Check sheet for the modelled part. Datum: model origin and axes. Units: mm. Face numbers are marked on the shaded views. A direction names the side the tool comes from. Round coordinates to 2 decimals unless told otherwise and drop trailing zeros. Write each loop counter-clockwise with the first axis right and the second up, starting at its lowest first coordinate (ties: lowest second). Pieces come first, ordered by that corner, then holes. Notation, with made-up numbers: (-21, -16.5) -> (31, -16.5) arc R36 cw to (31, 18.5) -> close; hole circle Ø11 at (18.5, 81). An arc over 180 degrees is marked (long way). Write item = value, one per line.
from build123d import *

# Parameters (mm, degrees)
SKETCH1_W           = 177.8
SKETCH1_H           = 50.8
BOSS_EXTRUDE2_DEPTH = 101.6
SKETCH5_W           = 101.6
SKETCH5_H           = 50.8
BOSS_EXTRUDE3_DEPTH = 76.2
BOSS_EXTRUDE4_DEPTH = 50.8
BOSS_EXTRUDE5_REACH = 103.6
SKETCH6_W           = 101.6
SKETCH6_H           = 50.8


with BuildPart() as part:
    # Sketch1 → Boss-Extrude2 (new body)
    with BuildSketch(Plane.XY):
        with Locations((88.9, 25.4)):
            Rectangle(SKETCH1_W, SKETCH1_H)
    extrude(amount=-BOSS_EXTRUDE2_DEPTH)

    # Sketch5 → Boss-Extrude3 (add)
    with BuildSketch(Plane(origin=(0, 0, 0), x_dir=(0, 0, -1), z_dir=(1, 0, 0))):
        with Locations((50.8, 76.2)):
            Rectangle(SKETCH5_W, SKETCH5_H)
    extrude(amount=BOSS_EXTRUDE3_DEPTH)

    # Sketch4 → Boss-Extrude4 (add)
    with BuildSketch(Plane(origin=(0, 50.8, 0), x_dir=(1, 0, 0), z_dir=(0, 1, 0))):
        Polygon((76.2, 50.8), (76.2, 0), (177.8, 50.8), (177.8, 101.6), (177.395806452, 101.6), (177.395806452, 50.8), align=None)
    extrude(amount=BOSS_EXTRUDE4_DEPTH)

    # Sketch6 → Boss-Extrude5 (add, up to next)
    with BuildSketch(Plane(origin=(76.2, 101.6, -101.6), x_dir=(1, 0, 0), z_dir=(0, 0, 1)), mode=Mode.PRIVATE) as boss_extrude5_sk1:
        with Locations((50.8, -25.4)):
            Rectangle(SKETCH6_W, SKETCH6_H)
    boss_extrude5_tool1 = extrude(boss_extrude5_sk1.sketch, amount=BOSS_EXTRUDE5_REACH, mode=Mode.PRIVATE) - part.part
    add(boss_extrude5_tool1.solids().sort_by_distance((127, 76.2, -101.6))[0])


solid = part.part
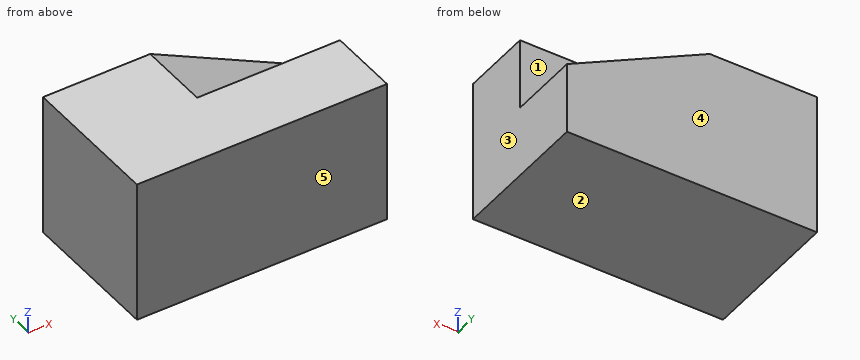
(1) Release check for a two-part mould opening along Y. For the marked faces 3, 4 and 5 record: pulls with the +Y half, pulls with the -Y half, needs draft (parallel to the pull), parting line crosses it, or undercut.
Worked answers:
face_3 = needs draft
face_4 = pulls with the +Y half
face_5 = pulls with the -Y half
(2) Sectioned sample at C-C on y = 82. Enter the section's corners in (x, z), then the cut area to 3 significant figures.
Worked answers:
outline = (0, -101.6) -> (177.8, -101.6) -> (177.8, -50.8) -> (76.2, 0) -> (0, 0) -> close
area = 15,500 mm²
(3) Material ranges on L1, parallel to Z at x = 169, y = 91.5; L2, parallel to Z at x = 114, y = 95.5; L3, parallel to X at y = 88, z = -28.5, recorded low to high. Write a range as [from, to].
Worked answers:
L1 = [-101.6, -46.4]
L2 = [-101.6, -18.9]
L3 = [0, 133.2]
(4) Sectioned sample at A-A on z = -41.5. Enter the section's corners in (x, y), then the cut area to 3 significant figures.
Worked answers:
outline = (0, 0) -> (177.8, 0) -> (177.8, 50.8) -> (159.2, 50.8) -> (159.2, 101.6) -> (0, 101.6) -> close
area = 17,100 mm²
(5) Sectioned sample at B-B on x = 141.5. Enter the section's corners in (y, z).
Worked answers:
outline = (0, -101.6) -> (101.6, -101.6) -> (101.6, -32.65) -> (50.8, -32.65) -> (50.8, 0) -> (0, 0) -> close
(6) Go/stop test with flat-tipped pins: P1, Ø1.5, axis at x = 159, z = -82, coming from the -Y side; P2, Ø3, axis at x = 145, z = -10.5, coming from the +Y side. Record where each tip stops, or that it passes through.
Worked answers:
P1 = 0
P2 = 50.8
(7) Access from +Z, -Z, +X, -X, +Y, -Y to the whole of each face (thin tool, end or side, straight path). Record for the marked faces 1 and 2.
Worked answers:
face_1 = +Z, +X, +Y
face_2 = -Z, +X, -X, +Y, -Y
